Build history of the part. All positions in model axes, mm. Coordinates: 2 decimals unless noted, no trailing zeros. Order: outer loops, then holes, each group sorted by start corner. A loop starts at its lowest first (then second) coordinate and runs counter-clockwise, first axis right, second up. Notation, with made-up numbers: M -31.75,0.25 L -5.75,0.25 A14 cw -5.75,19.25 Z; hole C -35.5,51 d11. An arc over 180 degrees is marked long. Write item = value, one per line. Start each with the question number.
Q1. Drill centre lines: probe 1 along X at (y, z) = (0.2, -1.15); probe 2 along X at (y, z) = (-0.8, -0.3); probe 3 along Z at (x, y) = (4.75, 0.4). Where is each one in solid material? Low to high.
Q2. Pull direction Y, two halves, no side cores. Call faces 1 (the face through (-0.109, 0.043, -0.014)), 2 (the face through (-0.203, 1.617, 0.67)), 3 (the face through (8, 0, 0)): released by +Y, released by -Y, zero draft, split by the parting line, or undercut.
Q3. Band-saw the part on A-A on x = 6.5. Write the cut outline in (y, z).
Q4. Pin check, flat tips, straight feed: P1, Ø1, axis at x = 5, y = 0, coming from the -Z side; P2, Ø1.5, axis at x = 7, z = 1, coming from the -Y side; P3, Ø2, axis at x = 4.5, z = 1.5, coming from the +Y side. Stop position of each tip, or through.
Autodesk Inventor part; units mm, degrees
ref_plane "Work Plane1" through (29, 0, 0) normal (0, -1, 0) x (1, 0, 0)
ref_plane "YZ Plane" through (0, 0, 0) normal (1, 0, 0) x (0, 1, 0)
ref_plane "XZ Plane" through (0, 0, 0) normal (0, 1, 0) x (-1, 0, 0)
sketch "Sketch1" plane through (0, 0, 0) normal (0, 0, 1) x (1, 0, 0)
  line L0 (-0.0833, 0) -> (8, 0)
  line L1 (8, 0) -> (8, 1)
  line L2 (8, 1) -> (5, 1)
  line L3 (5, 1) -> (4.6932, 1)
  line L4 (4.6932, 1) -> (0, 1)
  line L5 (0, 1) -> (0, 1.75)
  line L6 (0, 1.75) -> (-1.2, 1.75)
  line L7 (-1.2, 1.75) -> (-1.2, 0.7217)
  line L8 (-1.2, 0.7217) -> (-0.5, 0.7217)
  line L9 (-0.5, 0.7217) -> (-0.0833, 0)
  line L10 (-3.04, 0) -> (9.84, 0)
  line L11 (0, -0.35) -> (0, 2.1)
  line L12 (5, 1) -> (0, 1) construction
  dimension "d1" = 3
  dimension "d2" = 0.3068
  dimension "d3" = 1.2
  dimension "d4" = 0.7
  dimension "d5" = 60
  dimension "d6" = 2
  dimension "d7" = 2
  dimension "d8" = 1.4434
  dimension "d9" = 3.5
  dimension "d26" = 8
revolve "Body" add sketch "Sketch1" angle 360 about axis through (-0.0833, 0, 0) along (1, 0, 0)
sketch "Sketch2" plane through (-1.2, 0, 0) normal (-1, 0, 0) x (0, 0, 1)
  circle A0 centre (0, 0) radius 0.7217
  line L0 (0, -2.45) -> (0, 2.45)
  line L1 (-2.45, 0) -> (2.45, 0)
  line L2 (0.7217, 0) -> (0.3608, -0.625)
  line L3 (0.3608, -0.625) -> (-0.3608, -0.625)
  line L4 (-0.3608, -0.625) -> (-0.7217, 0)
  line L5 (-0.7217, 0) -> (-0.3608, 0.625)
  line L6 (-0.3608, 0.625) -> (0.3608, 0.625)
  line L7 (0.3608, 0.625) -> (0.7217, 0)
extrude "Slot" add sketch "Sketch2" against normal up to next contours L7 A0 | A0 L2 | L6 L0 A0 | A0 L0 L3 | L0 L6 A0 | A0 L3 L0 | L4 A0 | A0 L5
fillet "Fillet1" radius 0.8 1 edges at (-1.2, -1.75, 0)
chamfer "Chamfer1" distance 0.3067 distance2 0.3067 1 edges at (8, -1, 0) measured on face at (8, -0.479, -0.3842)
ref_plane "Work Plane1" through (29, 0, 0) normal (0, -1, 0) x (1, 0, 0)
fillet "Fillet2" radius 0.1 1 edges at (0, -1, 0)
thread "Thread2"
equation "\"d15\" = -0.5 * SPD + 0.5 * GD"
equation "\"d16\" = GUL"
equation "\"GD\" = NND"
equation "\"NLG\" = 6"
equation "\"GEL\" = 4.5"
equation "\"KOD\" = 5.7"
equation "\"KOH\" = 1.65"
equation "\"INTI\" = 1.04"
equation "\"GAL\" = 0.61345 * PTC"
equation "\"GUL\" = 0.61345 * PTC"
equation "\"BDM\" = NND"
equation "\"SW\" = 2"
equation "\"RR\" = 1.45"
equation "\"SPD\" = NND - 1.2269 * PTC"
equation "\"R\" = 0.3"
equation "\"TOA\" = 30deg"
equation "\"GD1\" = THREADDIA - 1.2269 * PTC"
equation "\"THREADDIA\" = 3"
equation "\"PTC\" = 0.5"
equation "\"NND\" = 3"
equation "\"KOH1\" = 0.2"
equation "\"E0\" = 2.303"
properties part number "M2x8 Bolt" material "Stainless Steel"
Recorded:
q1.probe_1 = -1.17 to 0
q1.probe_2 = -1.2 to 7.84
q1.probe_3 = -0.92 to 0.92
q2.face_1 = undercut
q2.face_2 = split by the parting line
q2.face_3 = zero draft
q3.outline = C 0,0 d2
q4.P1 = -1
q4.P2 = -0.97
q4.P3 = 0.87
